Input: part model. Units: mm. Frame: model coordinates. A direction names the side the tool comes from. Give positions to 0.01 mm unless a question says otherwise; leave off trailing zeros. Write each loop counter-clockwise with the first axis right and the second up, starting at its lowest first coordinate (ties: lowest second). Pieces come first, ordered by that corner, then holes. Notation, with made-up numbers: (11.5, -8.75) - (50.5, -8.75) arc R23 cw to (50.5, 9.25) - close; hole circle Ø9 at (-7.5, 11.5). An arc over 180 degrees is marked (long way). Answer as a JSON object with one key per item and string values. Group by question number.
from build123d import *

# Parameters (mm, degrees)
ESBO_O1_W                = 200
ESBO_O1_H                = 200
RESSALTO_EXTRUS_O1_DEPTH = 6
ESBO_O2_W                = 30
ESBO_O2_H                = 6
ESBO_O2_W_2              = 6
ESBO_O2_H_2              = 30
CORTE_EXTRUS_O1_DEPTH    = 10


with BuildPart() as part:
    # Esboço1 → Ressalto-extrusão1 (new body)
    with BuildSketch(Plane(origin=(0, 0, 0), x_dir=(1, 0, 0), z_dir=(0, 1, 0))):
        Rectangle(ESBO_O1_W, ESBO_O1_H)
    extrude(amount=RESSALTO_EXTRUS_O1_DEPTH)

    # Esboço2 → Corte-extrusão1 (cut)
    with BuildSketch(Plane(origin=(0, 6, 0), x_dir=(1, 0, 0), z_dir=(0, 1, 0))):
        with Locations((-55, -97)):
            Rectangle(ESBO_O2_W, ESBO_O2_H)
        with Locations((55, -97)):
            Rectangle(ESBO_O2_W, ESBO_O2_H)
        with Locations((-55, 97)):
            Rectangle(ESBO_O2_W, ESBO_O2_H)
        with Locations((55, 97)):
            Rectangle(ESBO_O2_W, ESBO_O2_H)
        with Locations((-97, 55)):
            Rectangle(ESBO_O2_W_2, ESBO_O2_H_2)
        with Locations((-97, -55)):
            Rectangle(ESBO_O2_W_2, ESBO_O2_H_2)
    extrude(amount=-CORTE_EXTRUS_O1_DEPTH, mode=Mode.SUBTRACT)


solid = part.part
1) Cut plane A-A on y = 1.6. Return the cut outline in (x, z), and give its area (3 significant figures).
2) Mould query, pull axis Z, two halves, no side actions, for faces 6 (the face through (-97, 3, 40)), 7 (the face through (-85, 3, 100)), 8 (the face through (-97, 3, -70)), 9 (the face through (40, 3, -97)). Classes: +Z half, -Z half, draft (parallel to the pull), parting line (faces both ways), or undercut.
3) Cut plane B-B on x = -55.5. Return the cut outline in (y, z).
4) Reachability of faces 1 (the face through (100, 3, 1)), 2 (the face through (-97, 3, 70)), 3 (the face through (-1, 3, -100)), 4 (the face through (70, 3, 97)), 5 (the face through (70, 3, -97)) from +Z, -Z, +X, -X, +Y, -Y: full face, straight path, thin tool, end or side. Return the list, or none.
5) Cut plane C-C on z = -47.5. Return the cut outline in (x, y), and give its area (3 significant figures).
6) Pin query (flat end, axial travel): P1, Ø3, axis at y = 4.5, z = 48, coming from the -X side; P2, Ø3, axis at x = 56.5, y = 2.5, coming from the -Z side. Return the tip coordinate at first contact, or that it passes through.
7) Line query: line 1 along X through (y, z) = (5.35, 61); line 2 along Z through (x, y) = (58, 0.4). Output: solid intervals per line, ascending. Write a range as from..to.
Filled in:
{
 "1": {"outline": "(-100, -100) - (-70, -100) - (-70, -94) - (-40, -94) - (-40, -100) - (40, -100) - (40, -94) - (70, -94) - (70, -100) - (100, -100) - (100, 100) - (70, 100) - (70, 94) - (40, 94) - (40, 100) - (-40, 100) - (-40, 94) - (-70, 94) - (-70, 100) - (-100, 100) - (-100, 70) - (-94, 70) - (-94, 40) - (-100, 40) - (-100, -40) - (-94, -40) - (-94, -70) - (-100, -70) - close", "area": "38,900 mm²"},
 "2": {"face 6": "undercut", "face 7": "+Z half", "face 8": "undercut", "face 9": "draft"},
 "3": {"outline": "(0, -94) - (6, -94) - (6, 94) - (0, 94) - close"},
 "4": {"face 1": "+Z, -Z, +X, +Y, -Y", "face 2": "-X, +Y, -Y", "face 3": "-Z, +X, -X, +Y, -Y", "face 4": "+Z, +Y, -Y", "face 5": "-Z, +Y, -Y"},
 "5": {"outline": "(-94, 0) - (100, 0) - (100, 6) - (-94, 6) - close", "area": "1,160 mm²"},
 "6": {"P1": "stops at x = -94", "P2": "stops at z = -94"},
 "7": {"line 1": "x = -94..100", "line 2": "z = -94..94"}
}
